For this review, take the finished solid that the model builds, in its own axes (mm). A direction names the side the tool comes from. Coordinates: 2 decimals unless noted, no trailing zeros. Loops run counter-clockwise (first coordinate to the right, second up) from the corner with the lowest first, then second, coordinate; pieces in that order, holes last. Notation, with made-up numbers: M 54.5,-10 L 91.5,-10 A22 cw 91.5,17 Z; hole C -1.75,10 d7. An arc over 180 degrees is marked long. Answer as a JSON object with one key per item and string values. Group by question number.
Item 1: Wall thickness on L1, parallel to Y at x = 31, z = 20; L2, parallel to X at y = 152.4, z = 53.5 (3 decimals); L3, parallel to Y at x = 93.5, z = 13.5: over which ranges is each line inside the solid? List them lowest first. Write a range as from..to.
Item 2: Add section B-B (y = 114.3). State the section outline as (x, z) points (3 decimals), then the cut area to 3 significant figures.
Item 3: Add section C-C (z = 10.5). Count the separate pieces of the cut face and the enclosed holes in it, then the cut area to 3 significant figures.
Item 4: Insertion check: pin 1 (20.5 mm diameter, centred on x = 96, y = 190, fed in from +Z); pin 2 (5 mm diameter, centred on x = 65, z = 32.5, fed in from -Y). Each pin has a flat end and moves straight along its axis. Give the tip position at first contact, or say it passes through.
Item 5: Tool access review of faces 1 (the face through (63, 119, 0)), 2 (the face through (63, 72.898, 51)), 3 (the face through (101, 196, 76.454)): name each direction out of +Z, -Z, +X, -X, +Y, -Y from which nothing blocks a thin tool from reaching the whole face with its end or side.
Item 6: Add section A-A (x = 31.75). State the section outline as (y, z) points (3 decimals).
Item 7: Mouldability with a two-part tool opening along X and no side actions: class faces 4 (the face through (41.266, 152.819, 33.793)), 5 (the face through (33.815, 28.675, 9.517)), 6 (the face through (127, 148, 39)), 7 (the face through (63, 158, 79.502)) as +X half, -X half, draft (parallel to the pull), parting line (faces both ways), or undercut.
from build123d import *

# Parameters (mm, degrees)
F0_W           = 127
F0_H           = 22.352
F1_DEPTH       = 241.3
F2_W           = 127
F2_H           = 168.402
F3_DEPTH       = 57.15
F5_D           = 19.05
F5_CSINK_D     = 38.1
F5_CSINK_ANGLE = 82
F6_D           = 19.05
F6_START       = 57.15
F6_CBORE_D     = 40.64
F6_CBORE_DEPTH = 3.048
F7_T1_DEPTH    = 149.352
F8_T1_DEPTH    = 88.9
F9_T1_DEPTH    = 88.9
F10_T1_DEPTH   = 149.352
F11_T1_DEPTH   = 143.002
F12_T1_DEPTH   = 143.002


# Not quite as in the source:
# - a fillet or chamfer that OpenCascade refuses, or shapes differently, is made with other operations: its cross-section is extruded or revolved along the edge and cut away or added


with BuildPart() as f1:
    # F0 (on Front) → F1 (new body)
    with BuildSketch(Plane.XZ):
        with Locations((63.5, 11.176)):
            Rectangle(F0_W, F0_H)
    extrude(amount=-F1_DEPTH)

    # F2 (on face) → F3 (join)
    with BuildSketch(Plane.XY.offset(22.352)):
        with Locations((63.5, 157.099)):
            Rectangle(F2_W, F2_H)
    extrude(amount=F3_DEPTH)

    # F5 (through all)
    with Locations(Plane.XY.offset(79.502)):
        with Locations((31.75, 152.4), (92.075, 114.3)):
            CounterSinkHole(F5_D / 2, F5_CSINK_D / 2, counter_sink_angle=F5_CSINK_ANGLE)

    # F6 (through all)
    # its depths count from where the whole tool has entered the part; down to there all is cleared
    with Locations(Plane.XY.offset(79.502)):
        with Locations((92.075, 200.025, 0), (31.75, 37.973, -F6_START)):
            CounterBoreHole(F6_D / 2, F6_CBORE_D / 2, F6_CBORE_DEPTH)

    # F7: fillet of radius 25.4 on 1 edges, made by hand

    # F7_s2 → F7_t1 (cut)
    with BuildSketch(Plane.XY.offset(-63.5)):
        with BuildLine():
            add(Edge.make_bspline(
                [(101.6, 0), (127, 0), (127, 25.4)],
                knots=[0, 0, 0, 1, 1, 1], degree=2, weights=[1, 1, 1]))
            Line((127, 25.4), (127, 0))
            Line((127, 0), (101.6, 0))
        make_face()
    extrude(amount=F7_T1_DEPTH, mode=Mode.SUBTRACT)

    # F8: fillet of radius 12.7 on 1 edges, made by hand

    # F8_s2 → F8_t1 (cut)
    with BuildSketch(Plane.XY.offset(22.352)):
        with BuildLine():
            add(Edge.make_bspline(
                [(114.3, 72.898), (127, 72.898), (127, 85.598)],
                knots=[0, 0, 0, 1, 1, 1], degree=2, weights=[1, 1, 1]))
            Line((127, 85.598), (127, 72.898))
            Line((127, 72.898), (114.3, 72.898))
        make_face()
    extrude(amount=F8_T1_DEPTH, mode=Mode.SUBTRACT)

    # F9: fillet of radius 12.7 on 1 edges, made by hand

    # F9_s2 → F9_t1 (cut)
    with BuildSketch(Plane.XY.offset(22.352)):
        with BuildLine():
            add(Edge.make_bspline(
                [(0, 85.598), (0, 72.898), (12.7, 72.898)],
                knots=[0, 0, 0, 1, 1, 1], degree=2, weights=[1, 1, 1]))
            Line((12.7, 72.898), (0, 72.898))
            Line((0, 72.898), (0, 85.598))
        make_face()
    extrude(amount=F9_T1_DEPTH, mode=Mode.SUBTRACT)

    # F10: fillet of radius 25.4 on 1 edges, made by hand

    # F10_s2 → F10_t1 (cut)
    with BuildSketch(Plane.XY.offset(-63.5)):
        with BuildLine():
            add(Edge.make_bspline(
                [(0, 25.4), (0, 0), (25.4, 0)],
                knots=[0, 0, 0, 1, 1, 1], degree=2, weights=[1, 1, 1]))
            Line((25.4, 0), (0, 0))
            Line((0, 0), (0, 25.4))
        make_face()
    extrude(amount=F10_T1_DEPTH, mode=Mode.SUBTRACT)

    # F11: fillet of radius 12.7 on 1 edges, made by hand

    # F11_s2 → F11_t1 (cut)
    with BuildSketch(Plane.XY.offset(-31.75)):
        with BuildLine():
            add(Edge.make_bspline(
                [(114.3, 241.3), (127, 241.3), (127, 228.6)],
                knots=[0, 0, 0, 1, 1, 1], degree=2, weights=[1, 1, 1]))
            Line((127, 228.6), (127, 241.3))
            Line((127, 241.3), (114.3, 241.3))
        make_face()
    extrude(amount=F11_T1_DEPTH, mode=Mode.SUBTRACT)

    # F12: fillet of radius 12.7 on 1 edges, made by hand

    # F12_s2 → F12_t1 (cut)
    with BuildSketch(Plane.XY.offset(-31.75)):
        with BuildLine():
            add(Edge.make_bspline(
                [(0, 228.6), (0, 241.3), (12.7, 241.3)],
                knots=[0, 0, 0, 1, 1, 1], degree=2, weights=[1, 1, 1]))
            Line((12.7, 241.3), (0, 241.3))
            Line((0, 241.3), (0, 228.6))
        make_face()
    extrude(amount=F12_T1_DEPTH, mode=Mode.SUBTRACT)


solid = f1.part
From the geometry:
{
 "1": {"L1": "y = 0..17.67, 58.28..142.9, 161.9..241.3", "L2": "x = 0..22.225, 41.275..127", "L3": "y = 0..104.88, 123.72..190.61, 209.44..241.3"},
 "2": {"outline": "M 0,0 L 82.55,0 L 82.55,68.545 L 73.025,79.502 L 0,79.502 Z; M 101.6,0 L 127,0 L 127,79.502 L 111.125,79.502 L 101.6,68.545 Z", "area": "8,480 mm²"},
 "3": {"separate pieces": "1", "enclosed holes": "4", "area": "29,200 mm²"},
 "4": {"pin 1": "stops at z = 79.5", "pin 2": "stops at y = 72.9"},
 "5": {"face 1": "-Z, +X, -X, +Y, -Y", "face 2": "+Z, +X, -X, -Y", "face 3": "+Z"},
 "6": {"outline": "M 0,0 L 28.448,0 L 28.448,19.304 L 17.653,19.304 L 17.653,22.352 L 0,22.352 Z; M 47.498,0 L 142.875,0 L 142.875,68.545 L 133.35,79.502 L 72.898,79.502 L 72.898,22.352 L 58.293,22.352 L 58.293,19.304 L 47.498,19.304 Z; M 161.925,0 L 241.3,0 L 241.3,79.502 L 171.45,79.502 L 161.925,68.545 Z"},
 "7": {"face 4": "undercut", "face 5": "undercut", "face 6": "+X half", "face 7": "draft"}
}
